Build history of the part. All positions in model axes, mm. Face numbers are marked on the shaded views. A direction names the side the tool comes from. Round coordinates to 2 decimals unless told otherwise and drop trailing zeros. Write each loop counter-clockwise with the first axis right and the second up, starting at its lowest first coordinate (ties: lowest second). Pieces come first, ordered by that corner, then holes. Notation, with made-up numbers: M 75,6 L 111,6 A17 ccw 111,37 Z; hole C 6.25,47.25 d3. An arc over 180 degrees is marked long. Write item = value, one per line. Start each with the question number.
Q1. Probe L1, parallel to Z at x = -20, y = -37.75; L2, parallel to Y at x = -16.5, z = 8; L3, parallel to X at y = -24, z = 23. List the from-to ranges inside material, lowest first.
Q2. Band-saw the part on C-C on y = -27. State how many separate pieces and enclosed holes the cut face has, plus the area to 3 significant figures.
Q3. Drop flat-ended pins along their axis: P1, Ø8.5, axis at x = -7, y = -28.65, coming from the +Z side; P2, Ø10, axis at y = -28, z = 66, coming from the +X side; P3, Ø2, axis at y = -34.5, z = 52, coming from the +X side. Give the stop position or say it passes through.
Q4. Band-saw the part on A-A on x = -28.5. Write the cut outline in (y, z).
Q5. Pull direction Y, two halves, no side cores. Call the marked faces 6, 7 and 8: released by +Y, released by -Y, zero draft, split by the parting line, or undercut.
Q6. Tool access for the marked faces 1, 2, 3, 4 and 5: list every direction of +Z, -Z, +X, -X, +Y, -Y with a clear straight run to the whole face (end or side of a thin tool).
Q7. Band-saw the part on B-B on x = -16. Write the cut outline in (y, z), plus the area to 3 significant figures.
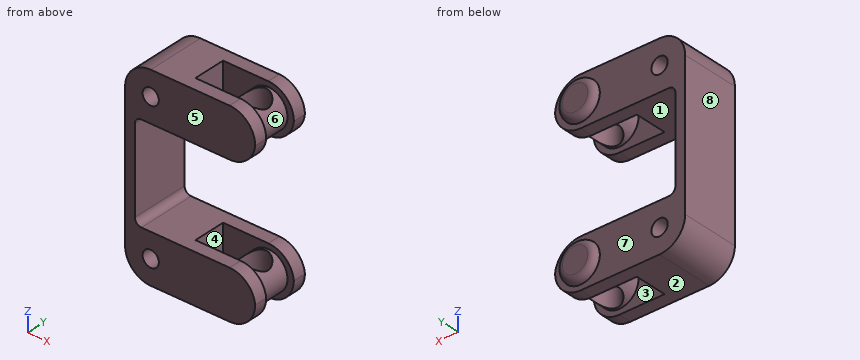
```python
from build123d import *

# Parameters (mm, degrees)
BOSS_EXTRUDE4_DEPTH = 76.2
FILLET1_R           = 10
SKETCH8_W           = 46.99
SKETCH8_H           = 38.1
CUT_EXTRUDE2_DEPTH  = 25.4
FILLET2_R           = 10
SKETCH9_R           = 7.493
BOSS_EXTRUDE5_DEPTH = 2.54
FILLET4_R           = 2.54
BOSS_EXTRUDE6_REACH = 94.231
SKETCH10_R          = 7.493
SKETCH11_R          = 5.334
CUT_EXTRUDE3_DEPTH  = 76.2
FILLET5_R           = 2.54
CUT_EXTRUDE5_REACH  = 94.824
SKETCH14_R          = 3.175


# Some blends are built 0.0001 mm under size
with BuildPart() as part:
    # Sketch7 → Boss-Extrude4 (new body)
    with BuildSketch(Plane.XY):
        Polygon((-47.824509335, -17.216733289), (2.975490665, -17.216733289), (2.975490665, -22.296733289), (-24.669160498, -22.296733289), (-24.669160498, -34.996733289), (2.975490665, -34.996733289), (2.975490665, -40.076733289), (-47.824509335, -40.076733289), (-47.824509335, -34.996733289), (-47.824509335, -22.296733289), align=None)
    extrude(amount=BOSS_EXTRUDE4_DEPTH)

    # Fillet1
    fillet1_edges = [part.edges().sort_by_distance(p)[0] for p in [
        (2.975490665, -19.756733289, 0),
        (2.975490665, -37.536733289, 0),
        (-47.824509335, -28.646733289, 0),
        (2.975490665, -37.536733289, 76.2),
        (2.975490665, -19.756733289, 76.2),
        (-47.824509335, -28.646733289, 76.2),
    ]]
    fillet(fillet1_edges, radius=FILLET1_R)

    # Sketch8 → Cut-Extrude2 (cut)
    with BuildSketch(Plane(origin=(0, -17.216733289, 0), x_dir=(1, 0, 0), z_dir=(0, 1, 0))):
        with Locations((-20.519509335, -38.1)):
            Rectangle(SKETCH8_W, SKETCH8_H)
    extrude(amount=-CUT_EXTRUDE2_DEPTH, mode=Mode.SUBTRACT)

    # Fillet2
    # the kernel refuses this fillet: 10 mm, written as the material it takes off along each edge
    with BuildSketch(Plane(origin=(2.975490665, -10.109801477, 57.15), x_dir=(-1, 0, 0), z_dir=(0, -1, 0)), Plane(origin=(2.975490665, 7.670198523, 57.15), x_dir=(-1, 0, 0), z_dir=(0, -1, 0))) as fillet2_piece_1:
        with BuildLine():
            CenterArc((9.954772725, -10), FILLET2_R, 90, 84.548680188)
            Line((0, -9.05), (-0.199095454, -9.031))
            ThreePointArc((-0.199095454, -9.031), (-0.2, -4.525), (-0.2, 0))
            Line((-0.2, 0), (0, 0.2))
            Line((0, 0.2), (9.954772725, 0.2))
            Line((9.954772725, 0.2), (9.954772725, 0))
        make_face()
    extrude(amount=54.853863623, mode=Mode.SUBTRACT)
    with BuildSketch(Plane(origin=(2.975490665, -10.109801477, 19.05), x_dir=(-1, 0, 0), z_dir=(0, -1, 0))) as fillet2_piece_2:
        with BuildLine():
            CenterArc((9.954772725, 10), FILLET2_R, 185.451319812, 84.548680188)
            Line((0, 9.05), (-0.199095454, 9.031))
            ThreePointArc((-0.199095454, 9.031), (-0.2, 4.525), (-0.2, 0))
            Line((-0.2, 0), (0, -0.2))
            Line((0, -0.2), (9.954772725, -0.2))
            Line((9.954772725, -0.2), (9.954772725, 0))
        make_face()
    extrude(amount=54.853863623, mode=Mode.SUBTRACT)
    with BuildSketch(Plane(origin=(2.975490665, 7.670198523, 19.05), x_dir=(0, 0, -1), z_dir=(0, -1, 0))) as fillet2_piece_3:
        with BuildLine():
            CenterArc((10, -9.954772725), FILLET2_R, 95.451319812, 84.548680188)
            Line((0, -9.954772725), (-0.2, -9.954772725))
            Line((-0.2, -9.954772725), (-0.2, 0))
            Line((-0.2, 0), (0, 0.2))
            ThreePointArc((0, 0.2), (4.525, 0.2), (9.031, 0.199095454))
            Line((9.031, 0.199095454), (9.05, 0))
        make_face()
    extrude(amount=54.853863623, mode=Mode.SUBTRACT)

    # Sketch9 → Boss-Extrude5 (add)
    with BuildSketch(Plane(origin=(0, -17.216733289, 0), x_dir=(1, 0, 0), z_dir=(0, 1, 0))):
        with Locations(Location((-7.001895697, -66.675, 0), (0, 0, 270))):
            Circle(SKETCH9_R)
        with Locations(Location((-7.001895697, -9.525, 0), (0, 0, 270))):
            Circle(SKETCH9_R)
    extrude(amount=BOSS_EXTRUDE5_DEPTH)

    # Fillet4
    fillet4_edges = [part.edges().sort_by_distance(p)[0] for p in [
        (-7.001895697, -14.676733289, 59.182),
        (-7.001895697, -14.676733289, 2.032),
    ]]
    fillet(fillet4_edges, radius=FILLET4_R - 0.0001)  # a hair under: the kernel refuses the full size

    # Sketch10 → Boss-Extrude6 (add, up to next)
    with BuildSketch(Plane(origin=(0, -34.996733289, 0), x_dir=(1, 0, 0), z_dir=(0, 1, 0)), mode=Mode.PRIVATE) as boss_extrude6_sk1:
        with Locations(Location((-7.001895697, -66.675, 0), (0, 0, 90))):
            Circle(SKETCH10_R)
    boss_extrude6_tool1 = extrude(boss_extrude6_sk1.sketch, amount=BOSS_EXTRUDE6_REACH, mode=Mode.PRIVATE) - part.part
    # Sketch10 → Boss-Extrude6 (add, up to next)
    with BuildSketch(Plane(origin=(0, -34.996733289, 0), x_dir=(1, 0, 0), z_dir=(0, 1, 0)), mode=Mode.PRIVATE) as boss_extrude6_sk2:
        with Locations(Location((-7.001895697, -9.525, 0), (0, 0, 90))):
            Circle(SKETCH10_R)
    boss_extrude6_tool2 = extrude(boss_extrude6_sk2.sketch, amount=BOSS_EXTRUDE6_REACH, mode=Mode.PRIVATE) - part.part
    add(boss_extrude6_tool1.solids().sort_by_distance((-7.001896, -34.996733, 66.675))[0])
    add(boss_extrude6_tool2.solids().sort_by_distance((-7.001896, -34.996733, 9.525))[0])

    # Sketch11 → Cut-Extrude3 (cut)
    with BuildSketch(Plane.XY.offset(76.2)):
        with Locations(Location((-7.001895697, -28.646733289, 0), (0, 0, 90.00000003))):
            Circle(SKETCH11_R)
    extrude(amount=-CUT_EXTRUDE3_DEPTH, mode=Mode.SUBTRACT)

    # Fillet5
    fillet5_edges = [part.edges().sort_by_distance(p)[0] for p in [
        (-44.014509335, -28.646733289, 57.15),
        (-44.014509335, -28.646733289, 19.05),
    ]]
    fillet(fillet5_edges, radius=FILLET5_R)

    # Sketch14 → Cut-Extrude5 (cut, up to next)
    with BuildSketch(Plane(origin=(0, -17.216733289, 0), x_dir=(1, 0, 0), z_dir=(0, 1, 0)), mode=Mode.PRIVATE) as cut_extrude5_sk1:
        with Locations(Location((-37.824509335, -9.525, 0), (0, 0, 270))):
            Circle(SKETCH14_R)
    cut_extrude5_tool1 = extrude(cut_extrude5_sk1.sketch, amount=-CUT_EXTRUDE5_REACH, mode=Mode.PRIVATE) & part.part
    # Sketch14 → Cut-Extrude5 (cut, up to next)
    with BuildSketch(Plane(origin=(0, -17.216733289, 0), x_dir=(1, 0, 0), z_dir=(0, 1, 0)), mode=Mode.PRIVATE) as cut_extrude5_sk2:
        with Locations(Location((-37.824509335, -66.675, 0), (0, 0, 270))):
            Circle(SKETCH14_R)
    cut_extrude5_tool2 = extrude(cut_extrude5_sk2.sketch, amount=-CUT_EXTRUDE5_REACH, mode=Mode.PRIVATE) & part.part
    add(cut_extrude5_tool1.solids().sort_by_distance((-37.824509, -17.216733, 9.525))[0], mode=Mode.SUBTRACT)
    add(cut_extrude5_tool2.solids().sort_by_distance((-37.824509, -17.216733, 66.675))[0], mode=Mode.SUBTRACT)


solid = part.part
```
Conclusion:
q1.L1 = 0 to 19.05, 57.15 to 76.2
q1.L2 = -40.08 to -35, -22.3 to -17.22
q1.L3 = -47.82 to -44.01
q2.separate_pieces = 5
q2.enclosed_holes = 2
q2.area = 998 mm^2
q3.P1 = through
q3.P2 = 0.49
q3.P3 = -44.01
q4.outline = M -40.08,0 L -17.22,0 L -17.22,19.05 L -40.08,19.05 Z; M -40.08,57.15 L -17.22,57.15 L -17.22,76.2 L -40.08,76.2 Z
q5.face_6 = undercut
q5.face_7 = released by +Y
q5.face_8 = zero draft
q6.face_1 = +X, +Y, -Y
q6.face_2 = -Z, +X, -X, +Y, -Y
q6.face_3 = none
q6.face_4 = +Z, -Z
q6.face_5 = +Z, -Z, +X, -X, -Y
q7.outline = M -40.08,0 L -35,0 L -35,19.05 L -40.08,19.05 Z; M -40.08,57.15 L -35,57.15 L -35,76.2 L -40.08,76.2 Z; M -22.3,0 L -17.22,0 L -17.22,19.05 L -22.3,19.05 Z; M -22.3,57.15 L -17.22,57.15 L -17.22,76.2 L -22.3,76.2 Z
q7.area = 387 mm^2
